from build123d import *

# Parameters (mm, degrees)
F2_R = 1.8854618593
F3_R = 2.1718744825


with BuildPart() as f1:
    # F0 (on Front) → F1 (revolve)
    with BuildSketch(Plane.XZ):
        Polygon((-12.3239438981, 0), (0, 0), (0, 57.6760545373), (-3.450702643, 57.6760545373), (-12.3239438981, 33.2746505737), (-3.450702643, 20.2112654741), align=None)
    revolve(axis=Axis((0, 0, 28.8380272686), (0, 0, -1)))

    # F2
    f2_edges = [f1.edges().sort_by_distance(p)[0] for p in [
        (12.323944, 0, 33.274651),
    ]]
    fillet(f2_edges, radius=F2_R)

    # F3
    f3_edges = [f1.edges().sort_by_distance(p)[0] for p in [
        (3.450703, 0, 20.211265),
        (12.323944, 0, 0),
        (-7.887323, 0, 10.105633),
    ]]
    fillet(f3_edges, radius=F3_R)

    # F4 (on Front) → F5 (revolve)
    with BuildSketch(Plane.XZ):
        with BuildLine():
            add(Edge.make_bspline(
                [(0, 55.6588992476), (-1.9346006023, 55.4044221137), (-5.9728011334, 55.2906711058), (-10.6749403377, 55.6049072132), (-13.2927423914, 56.5220602196)],
                knots=[0, 0, 0, 0, 0.469506717, 1, 1, 1, 1], degree=3))
            Line((0, 55.6588992476), (-1.8686421681, 60.7309341431))
            Line((-1.8686421681, 60.7309341431), (-13.2927423914, 56.5220602196))
        make_face()
    revolve(axis=Axis((-0.9343210841, 0, 58.1949166954), (0.3457049895, 0, -0.9383432529)))


solid = f1.part
Read the model definition and answer for the solid it produces. Units are mm, in the model's axes. Give positions to 0.01 mm unless a question says otherwise; leave off trailing zeros. Answer as CSV lines item,"result". Start each with the question number.
1) Find section A-A (x = 7). State how many separate pieces and enclosed holes the cut face has, then the cut area to 3 significant figures.
2) Straight lines are drawn through the part: L1, parallel to Z at x = -4.5, y = -7; L2, parallel to Z at x = -6.75, y = -4.25; L3, parallel to Z at x = -10, y = 5.5. For each, find the intervals that lie inside material, in ascending order. Write a range as from..to.
3) Determine the mould class of faces 1 (the face through (-2.03, 0.17, 60.67)), 2 (the face through (-4.94, -2.048, 23.005)), 3 (the face through (0, 0, 0)) for opening direction Z: released by +Z, released by -Z, zero draft, split by the parting line, or undercut.
4) Each of these flat-tipped pins is pushed along its axis until it touches: pin 1 Ø2 at (y, z) = (0, 22) entering from -X; pin 2 Ø6 at (x, y) = (5, 2) entering from +Z; pin 3 Ø3 at (y, z) = (7.5, 28) entering from -X. Where does it stop, or does it pass through?
Findings below:
1,separate pieces,"3"
1,enclosed holes,"0"
1,area,"460 mm^2"
2,L1,"0..9.12, 27.38..44.28, 56.96..59.76"
2,L2,"0..9.9, 26.87..45.23, 55.93..58.93"
2,L3,"31.93..35.78, 56.52..57.74"
3,face 1,"released by +Z"
3,face 2,"undercut"
3,face 3,"released by -Z"
4,pin 1,"x = -5.34"
4,pin 2,"z = 64.37"
4,pin 3,"x = -6.93"
